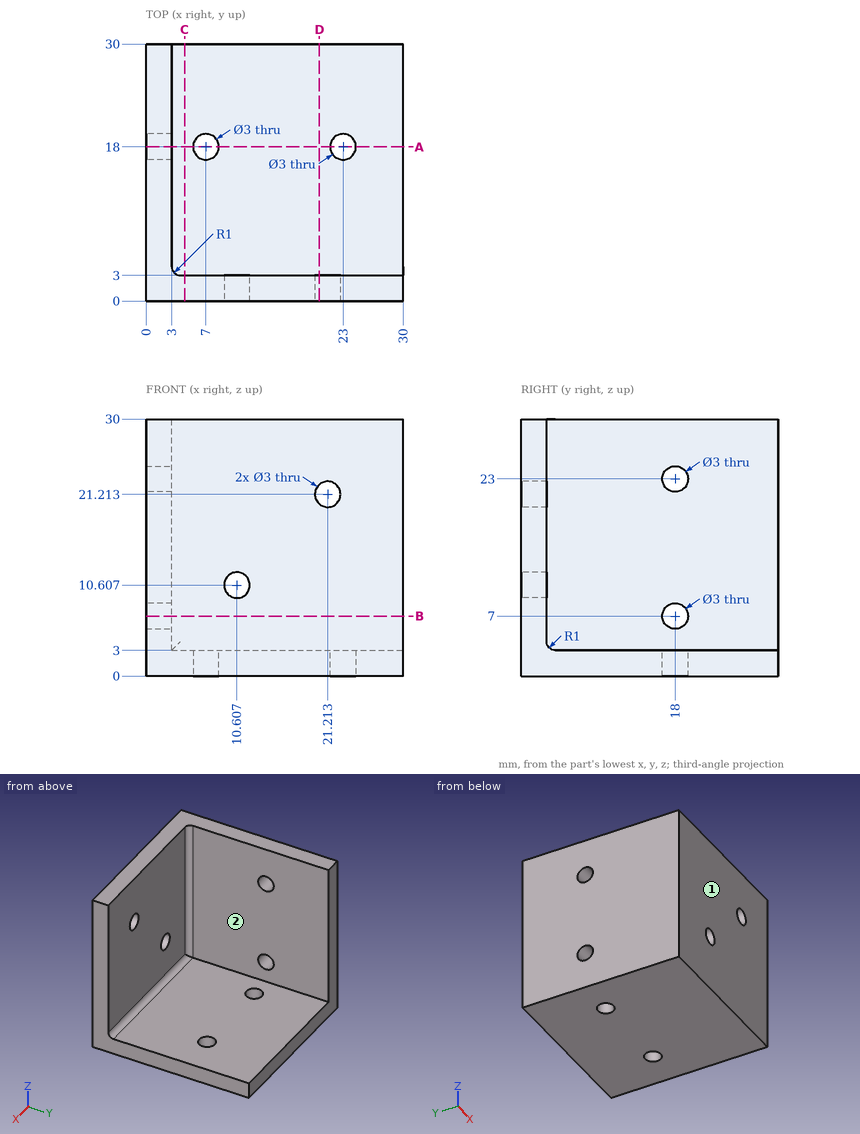
Design review of the part shown in the three views and the two pictorial views. Dimensions are in mm from the part's minimum x, y and z. A direction names the side the tool comes from. Round coordinates to 2 decimals unless told otherwise and drop trailing zeros. Loops run counter-clockwise (first coordinate to the right, second up) from the corner with the lowest first, then second, coordinate; pieces in that order, holes last. Notation, with made-up numbers: M 3,61.5 L 49,61.5 A24 ccw 49,74.5 Z; hole C -18.75,-10.5 d6. An arc over 180 degrees is marked long. Answer as a JSON object with one key per item and string values.
Item 1: Machinability: for the marked faces 1 and 2, which of the approach directions +Z, -Z, +X, -X, +Y, -Y give a long, thin tool a straight path to every point of the face, cutting with its end or side? Answer none if there is none.
Answer sheet:
{"face 1": "+Z, -Z, +X, -X, -Y", "face 2": "+Z, +X, +Y"}
Item 2: Clearance check with flat-ended pins moving along their axes: P1, Ø13, axis at x = 22, y = 20.5, coming from the +Z side; P2, Ø10, axis at y = 17, z = 25, coming from the +X side; P3, Ø4, axis at x = 10.61, z = 10.61, coming from the +Y side; P4, Ø2.5, axis at x = 21.21, z = 21.21, coming from the +Y side (3 decimals). State where each tip first meets the part, or that it passes through.
Answer sheet:
{"P1": "stops at z = 3", "P2": "stops at x = 3", "P3": "stops at y = 3", "P4": "passes through"}
Item 3: We need section B-B on z = 7. Give the boundary of the cut face in (x, y).
Answer sheet:
{"outline": "M 0,0 L 30,0 L 30,3 L 4,3 A1 cw 3,4 L 3,16.5 L 0,16.5 Z; M 0,19.5 L 3,19.5 L 3,30 L 0,30 Z"}
Item 4: We need section D-D on x = 20.25. Give the boundary of the cut face in (y, z), and give its area (3 significant figures).
Answer sheet:
{"outline": "M 0,0 L 30,0 L 30,3 L 4,3 A1 cw 3,4 L 3,20.06 L 0,20.06 Z; M 0,22.36 L 3,22.36 L 3,30 L 0,30 Z", "area": "164 mm^2"}
Item 5: We need section C-C on x = 4.5. Give the boundary of the cut face in (y, z), and give its area (3 significant figures).
Answer sheet:
{"outline": "M 0,0 L 30,0 L 30,3 L 4,3 A1 cw 3,4 L 3,30 L 0,30 Z", "area": "171 mm^2"}
Item 6: Wall thickness on L1, parallel to Y at x = 7, z = 0.7; L2, parallel to Y at x = 25, z = 27.75: over which ranges is each line inside the solid? List them lowest first. Write a range as from..to.
Answer sheet:
{"L1": "y = 0..16.5, 19.5..30", "L2": "y = 0..3"}
Item 7: We need section A-A on y = 18. Give the boundary of the cut face in (x, z).
Answer sheet:
{"outline": "M 0,0 L 5.5,0 L 5.5,3 L 3,3 L 3,5.5 L 0,5.5 Z; M 0,8.5 L 3,8.5 L 3,21.5 L 0,21.5 Z; M 0,24.5 L 3,24.5 L 3,30 L 0,30 Z; M 8.5,0 L 21.5,0 L 21.5,3 L 8.5,3 Z; M 24.5,0 L 30,0 L 30,3 L 24.5,3 Z"}
